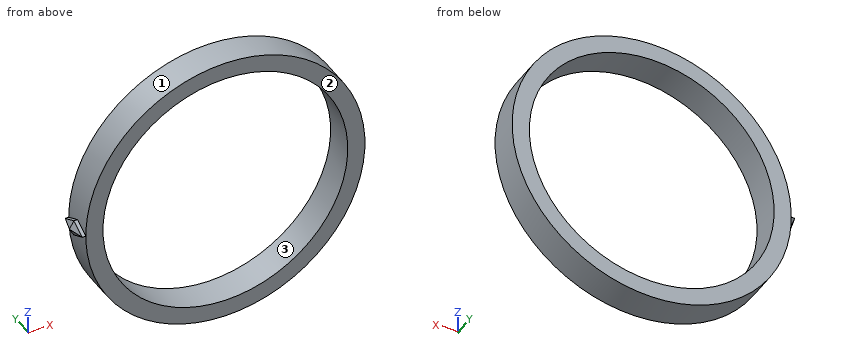
from build123d import *
from OCP.BRepFilletAPI import BRepFilletAPI_MakeChamfer

# Parameters (mm, degrees)
SKETCH1_R           = 19.5
SKETCH1_R_2         = 17.1
BOSS_EXTRUDE1_DEPTH = 4.347826087
BOSS_EXTRUDE2_DEPTH = 1.08695652
CHAMFER1_SIZE       = 0.6
CHAMFER1_SIZE2      = 0.971


with BuildPart() as part:
    # Sketch1 → Boss-Extrude1 (new body)
    with BuildSketch(Plane(origin=(0, 0, 0), x_dir=(1, 0, 0), z_dir=(0, 1, 0))):
        with Locations(Location((0, 0, 0), (0, 0, 270))):
            Circle(SKETCH1_R)
        with Locations(Location((0, 0, 0), (0, 0, 270))):
            Circle(SKETCH1_R_2, mode=Mode.SUBTRACT)
    extrude(amount=BOSS_EXTRUDE1_DEPTH)

    # Sketch2 → Boss-Extrude2 (add, symmetric)
    with BuildSketch(Plane.ZY.offset(19.5)):
        Polygon((0, 0.00928426), (-1.086956522, 2.173913043), (0, 4.338541827), (1.086956522, 2.173913043), align=None)
    extrude(amount=BOSS_EXTRUDE2_DEPTH, both=True)

    # Chamfer1: one chamfer whose edges measure the first distance from different faces: ONE call of the kernel's chamfer builder (chamfer() names one face for all edges)
    chamfer1_edges_1 = [part.edges().sort_by_distance(p)[0] for p in [
        (-20.58695652, 3.256227435, -0.543478261),
    ]]
    chamfer1_side_1 = [part.faces().sort_by_distance(p)[0] for p in [
        (-20.038389639, 3.251243161, -0.545981087),
    ]]
    chamfer1_edges_2 = [part.edges().sort_by_distance(p)[0] for p in [
        (-20.58695652, 1.091598652, -0.543478261),
    ]]
    chamfer1_side_2 = [part.faces().sort_by_distance(p)[0] for p in [
        (-20.038389639, 1.096582926, -0.545981087),
    ]]
    chamfer1_edges_3 = [part.edges().sort_by_distance(p)[0] for p in [
        (-20.58695652, 1.091598652, 0.543478261),
    ]]
    chamfer1_side_3 = [part.faces().sort_by_distance(p)[0] for p in [
        (-20.038389639, 1.096582926, 0.545981087),
    ]]
    chamfer1_edges_4 = [part.edges().sort_by_distance(p)[0] for p in [
        (-20.58695652, 3.256227435, 0.543478261),
    ]]
    chamfer1_side_4 = [part.faces().sort_by_distance(p)[0] for p in [
        (-20.038389639, 3.251243161, 0.545981087),
    ]]
    chamfer1 = BRepFilletAPI_MakeChamfer(part.part.solid().wrapped)
    for e in chamfer1_edges_1:
        chamfer1.Add(CHAMFER1_SIZE, CHAMFER1_SIZE2, e.wrapped, chamfer1_side_1[0].wrapped)  # the first distance lies on this face
    for e in chamfer1_edges_2:
        chamfer1.Add(CHAMFER1_SIZE, CHAMFER1_SIZE2, e.wrapped, chamfer1_side_2[0].wrapped)  # the first distance lies on this face
    for e in chamfer1_edges_3:
        chamfer1.Add(CHAMFER1_SIZE, CHAMFER1_SIZE2, e.wrapped, chamfer1_side_3[0].wrapped)  # the first distance lies on this face
    for e in chamfer1_edges_4:
        chamfer1.Add(CHAMFER1_SIZE, CHAMFER1_SIZE2, e.wrapped, chamfer1_side_4[0].wrapped)  # the first distance lies on this face
    add(Compound.cast(chamfer1.Shape()), mode=Mode.REPLACE)


solid = part.part
Part model, mm, in its own coordinate system. Face numbers are marked on the shaded views. Round coordinates to 2 decimals unless told otherwise and drop trailing zeros. Order: outer loops, then holes, each group sorted by start corner. A loop starts at its lowest first (then second) coordinate and runs counter-clockwise, first axis right, second up. Notation, with made-up numbers: (69, 39) -> (119, 39) arc R17 cw to (119, 60) -> close; hole circle Ø6 at (-17.5, 23). An arc over 180 degrees is marked (long way). Put each result on its own line as item: value.
Q1. Band-saw the part on A-A (x = 0). Give the cut face in (y, z), and give its area (3 significant figures).
From the geometry:
outline: (0, -19.5) -> (4.35, -19.5) -> (4.35, -17.1) -> (0, -17.1) -> close; (0, 17.1) -> (4.35, 17.1) -> (4.35, 19.5) -> (0, 19.5) -> close
area: 20.9 mm2
Q2. Pin check, flat tips, straight feed: pin 1 Ø2 at (y, z) = (3, -10) entering from +X; pin 2 Ø2 at (y, z) = (2.5, 8) entering from +X. Stop position of each tip, or through.
From the geometry:
pin 1: stops at x = 17.3
pin 2: stops at x = 18.2
Q3. Band-saw the part on B-B (z = -12). Give the cut face in (x, y).
From the geometry:
outline: (-15.37, 0) -> (-12.18, 0) -> (-12.18, 4.35) -> (-15.37, 4.35) -> close; (12.18, 0) -> (15.37, 0) -> (15.37, 4.35) -> (12.18, 4.35) -> close
Q4. Wall check: line 1 (X direction, y = 1.25, z = -15.5); line 2 (Z direction, x = -10, y = 1.45); line 3 (Z direction, x = 7.5, y = 2.8). Give the ranges that are in metal, low to high. Write a range as [from, to].
From the geometry:
line 1: x = [-11.83, -7.22], [7.22, 11.83]
line 2: z = [-16.74, -13.87], [13.87, 16.74]
line 3: z = [-18, -15.37], [15.37, 18]
Q5. Pull direction Z, two halves, no side cores. Call the marked faces 1, 2 and 3: pulls with the +Z half, pulls with the -Z half, needs draft (parallel to the pull), parting line crosses it, or undercut.
From the geometry:
face 1: parting line crosses it
face 2: needs draft
face 3: undercut
Q6. Band-saw the part on C-C (y = 3.3). Give the cut face in (x, z), and give its area (3 significant figures).
From the geometry:
outline: (-20.27, 0) -> (-19.99, -0.52) -> (-19.49, -0.52) arc R19.5 ccw (long way) to (-19.49, 0.52) -> (-19.99, 0.52) -> close; hole circle Ø34.2 at (0, 0)
area: 277 mm2
